```python
from build123d import *

# Parameters (mm, degrees)
F0_W           = 250
F0_H           = 183
F1_DEPTH       = 8
F3_D           = 4.4
F3_CBORE_D     = 8.25
F3_CBORE_DEPTH = 4
F4_D           = 18
F5_D           = 5


# Not quite as in the source:
# - a feature names something its author has since deleted; it is built from what else it names


with BuildPart() as f1:
    # F0 (on Top) → F1 (new body)
    with BuildSketch(Plane.XY):
        Rectangle(F0_W, F0_H)
    extrude(amount=F1_DEPTH)

    # F3 (through all)
    with Locations(Plane.XY.offset(8)):
        with Locations((-113, 68.5), (-113, -76.5), (113, -76.5), (113, 68.5), (71.5, 83.5), (-71.5, 83.5)):
            CounterBoreHole(F3_D / 2, F3_CBORE_D / 2, F3_CBORE_DEPTH)

    # F4 (through all)
    with Locations(Plane.XY.offset(8)):
        with Locations((15, -76.5)):
            Hole(F4_D / 2)

    # F5 (through all)
    with Locations(Plane.XY.offset(8)):
        with Locations((100, 58.5), (100, 33.5), (100, 8.5), (100, -16.5), (100, -41.5), (100, -66.5), (75, -66.5), (75, -41.5), (75, -16.5), (75, 8.5), (75, 33.5), (75, 58.5), (50, 58.5), (50, 33.5), (50, 8.5), (50, -16.5), (50, -41.5), (50, -66.5), (25, -66.5), (0, -66.5), (-25, -66.5), (-50, -66.5), (-75, -66.5), (-100, -66.5), (-100, -41.5), (-75, -41.5), (-50, -41.5), (-25, -41.5), (0, -41.5), (25, -41.5), (25, -16.5), (0, -16.5), (-25, -16.5), (-50, -16.5), (-75, -16.5), (-100, -16.5), (-100, 8.5), (-75, 8.5), (-50, 8.5), (-25, 8.5), (0, 8.5), (25, 8.5), (25, 33.5), (0, 33.5), (-25, 33.5), (-50, 33.5), (-75, 33.5), (-100, 33.5), (-100, 58.5), (-75, 58.5), (-50, 58.5), (25, 58.5), (-25, 58.5), (0, 58.5)):
            Hole(F5_D / 2)


solid = f1.part
```
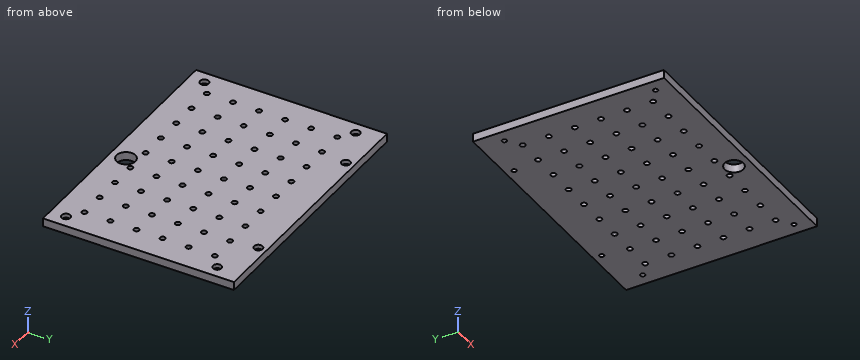
For this review, take the finished solid that the model builds, in its own axes (mm). Coordinates: 2 decimals unless noted, no trailing zeros. Order: outer loops, then holes, each group sorted by start corner. A loop starts at its lowest first (then second) coordinate and runs counter-clockwise, first axis right, second up. Notation, with made-up numbers: (85, -12.5) - (128, -12.5) arc R21 cw to (128, 21.5) - close; hole circle Ø7 at (-19, 43). An arc over 180 degrees is marked (long way). Answer as a JSON object with one key per item and string values. Group by question number.
1. We need section A-A on x = 15. State the section outline as (y, z) points, then the cut area to 3 significant figures.
2. We need section C-C on z = 5.25. Give the number of separate pieces and of enclosed holes in the cut face, then the cut area to 3 significant figures.
3. We need section B-B on x = -50. State the section outline as (y, z) points, then the cut area to 3 significant figures.
4. For probe 1 along X at (y, z) = (-74, 3.25); probe 2 along Y at (x, z) = (12, 5), list the stretches that pass through material, from the lowest coordinate up.
5. Clearance check with a flat-ended pin moving along its axis: P1, Ø3, axis at x = -75, y = -66.5, coming from the -Z side. State where the tip first meets the part, or that it passes through.
Final values:
{
 "1": {"outline": "(-91.5, 0) - (-85.5, 0) - (-85.5, 8) - (-91.5, 8) - close; (-67.5, 0) - (91.5, 0) - (91.5, 8) - (-67.5, 8) - close", "area": "1,320 mm²"},
 "2": {"separate pieces": "1", "enclosed holes": "61", "area": "44,100 mm²"},
 "3": {"outline": "(-91.5, 0) - (-69, 0) - (-69, 8) - (-91.5, 8) - close; (-64, 0) - (-44, 0) - (-44, 8) - (-64, 8) - close; (-39, 0) - (-19, 0) - (-19, 8) - (-39, 8) - close; (-14, 0) - (6, 0) - (6, 8) - (-14, 8) - close; (11, 0) - (31, 0) - (31, 8) - (11, 8) - close; (36, 0) - (56, 0) - (56, 8) - (36, 8) - close; (61, 0) - (91.5, 0) - (91.5, 8) - (61, 8) - close", "area": "1,220 mm²"},
 "4": {"probe 1": "-125 to 6.35, 23.65 to 125", "probe 2": "-91.5 to -84.99, -68.01 to 91.5"},
 "5": {"P1": "through"}
}
